Autodesk Inventor part; units mm, degrees
ref_plane "YZ Plane" through (0, 0, 0) normal (1, 0, 0) x (0, 1, 0)
ref_plane "XZ Plane" through (0, 0, 0) normal (0, 1, 0) x (-1, 0, 0)
ref_plane "XY Plane" through (0, 0, 0) normal (0, 0, 1) x (1, 0, 0)
sketch "Sketch1" plane through (0, 0, 0) normal (0, 0, 1) x (1, 0, 0)
  line L0 (0, 0) -> (-14.478, 0)
  line L1 (-14.478, 0) -> (-14.478, 2.54)
  line L2 (-14.478, 2.54) -> (-11.684, 2.54)
  line L3 (-11.684, 2.54) -> (-11.684, 7.62)
  line L4 (-11.684, 7.62) -> (-14.478, 7.62)
  line L5 (-14.478, 7.62) -> (-14.478, 15.24)
  line L6 (-14.478, 15.24) -> (-21.082, 15.24)
  line L7 (-21.082, 15.24) -> (-21.082, 18.034)
  line L8 (-21.082, 18.034) -> (-17.526, 18.034)
  line L9 (-17.526, 18.034) -> (-17.526, 20.828)
  line L10 (-17.526, 20.828) -> (0, 20.828)
  line L11 (0, 20.828) -> (0, 0)
  dimension "d0" = 17.526
  dimension "d1" = 21.082
  dimension "d2" = 14.478
  dimension "d3" = 11.684
  dimension "d4" = 2.794
  dimension "d5" = 5.588
  dimension "d7" = 18.288
  dimension "d8" = 13.208
  dimension "d9" = 20.828
revolve "Revolution1" add sketch "Sketch1" angle 360 about axis through (0, 20.828, 0) along (0, -1, 0)
chamfer "Chamfer1" distance 0.254 angle 45 1 edges at (14.478, 0, 0)
properties part number "GL45 bottle cap insert; solid"
Here's how the part is built. I have some questions about the finished solid (model axes, mm). A direction names the side the tool comes from. Give positions to 0.01 mm unless a question says otherwise; leave off trailing zeros. Write each loop counter-clockwise with the first axis right and the second up, starting at its lowest first coordinate (ties: lowest second). Pieces come first, ordered by that corner, then holes. Notation, with made-up numbers: (-33, -6) -> (-11, -6) arc R30 cw to (-11, 28) -> close; hole circle Ø8 at (-30, 6). An arc over 180 degrees is marked (long way). Use one line per item in the form item = value. Start each with the question number.
1. If I drill on L1, parallel to Y at x = 15, z = 11.5; L2, parallel to Y at x = -10.5, z = -9; L3, parallel to X at y = 11.5, z = -0.5, over which ranges is the centre line in solid material (lowest first)?
2. Thinking about a two-plate mould opening in Y: for faces 1 (the face through (10, 7.62, -7)), 2 (the face through (0, 20.828, 0)), 3 (the face through (-16.72, 19.45, 5.26)), which applies, +Y half, -Y half, draft (parallel to the pull), parting line (faces both ways), or undercut?
3. Imagine slicing it at B-B on x = 0. List the corners of the cut face in (y, z) for me, plus the area to 3 significant figures.
4. Imagine slicing it at D-D on y = 14. List the corners of the cut face in (x, z) for me.
5. Imagine slicing it at A-A on z = 0. List the corners of the cut face in (x, y) for me, plus the area to 3 significant figures.
6. On a 3-axis mill with a long thin cutter (end or side, diameter ignored), from which of +Z, -Z, +X, -X, +Y, -Y can I reach the whole of each face in a straight line? I mean faces 4 (the face through (-14, 15.24, -5)), 5 (the face through (8, 18.034, -16)), 6 (the face through (2.533, 5.116, -11.406)). Say none if no direction works.
7. Will these pins go through, and if not, where does the flat tip stop? pin 1 Ø4 at (x, y) = (13, 13.5) entering from -Z; pin 2 Ø6 at (x, y) = (-5.5, 15) entering from +Z; pin 3 Ø5 at (x, y) = (13, 17) entering from -Z.
8. Imagine slicing it at C-C on y = 17.25. List the corners of the cut face in (x, z) for me, plus the area to 3 significant figures.
Entries:
q1.L1 = 15.24 to 18.03
q1.L2 = 0 to 2.54, 7.62 to 20.83
q1.L3 = -14.47 to 14.47
q2.face_1 = undercut
q2.face_2 = +Y half
q2.face_3 = draft
q3.outline = (0, -14.22) -> (0.25, -14.48) -> (2.54, -14.48) -> (2.54, -11.68) -> (7.62, -11.68) -> (7.62, -14.48) -> (15.24, -14.48) -> (15.24, -21.08) -> (18.03, -21.08) -> (18.03, -17.53) -> (20.83, -17.53) -> (20.83, 17.53) -> (18.03, 17.53) -> (18.03, 21.08) -> (15.24, 21.08) -> (15.24, 14.48) -> (7.62, 14.48) -> (7.62, 11.68) -> (2.54, 11.68) -> (2.54, 14.48) -> (0.25, 14.48) -> (0, 14.22) -> close
q3.area = 629 mm²
q4.outline = circle Ø28.96 at (0, 0)
q5.outline = (-21.08, 15.24) -> (-14.48, 15.24) -> (-14.48, 7.62) -> (-11.68, 7.62) -> (-11.68, 2.54) -> (-14.48, 2.54) -> (-14.48, 0.25) -> (-14.22, 0) -> (14.22, 0) -> (14.48, 0.25) -> (14.48, 2.54) -> (11.68, 2.54) -> (11.68, 7.62) -> (14.48, 7.62) -> (14.48, 15.24) -> (21.08, 15.24) -> (21.08, 18.03) -> (17.53, 18.03) -> (17.53, 20.83) -> (-17.53, 20.83) -> (-17.53, 18.03) -> (-21.08, 18.03) -> close
q5.area = 629 mm²
q6.face_4 = -Y
q6.face_5 = +Y
q6.face_6 = none
q7.pin_1 = -17.32
q7.pin_2 = 20.93
q7.pin_3 = -18.28
q8.outline = circle Ø42.16 at (0, 0)
q8.area = 1,400 mm²
